Verification items for this drawing (mm, ordinates from the low corner). A direction names the side the tool comes from. Round coordinates to 2 decimals unless told otherwise and drop trailing zeros. Loops run counter-clockwise (first coordinate to the right, second up) from the corner with the lowest first, then second, coordinate; pieces in that order, holes last. Notation, with made-up numbers: M 69.5,57.5 L 88.5,57.5 A12 ccw 88.5,76.5 Z; hole C 84,10 d9. An arc over 180 degrees is marked long. Use one line per item in the form item = value. Start each with the question number.
1. Set-up check for the marked faces 4, 5 and 6: record each of +Z, -Z, +X, -X, +Y, -Y from which the full face is reachable in a straight line by a thin tool's end or side.
2. Material ranges on line 1 (Y direction, x = 16, z = 1) (3 decimals); line 2 (Y direction, x = 12, z = 1.5) (3 decimals); line 3 (X direction, y = 18, z = 2.8), recorded low to high.
3. Go/stop test with flat-tipped pins: pin 1 (0.9 mm diameter, centred on x = 4.5, z = 1, fed in from -Y) (3 decimals); pin 2 (1.6 mm diameter, centred on y = 2, z = 1.5, fed in from -X) (3 decimals); pin 3 (1.6 mm diameter, centred on y = 2, z = 2.5, fed in from +X) (3 decimals). Record where each tip stops, or that it passes through.
4. Cross-section at D-D (x = 5). Record the boundary of the cut face in (y, z) (3 decimals).
5. Draft check along X on the marked faces 1, 2 and 3. Enter one of: pulls with the +X half, pulls with the -X half, needs draft (parallel to the pull), parting line crosses it, or undercut.
6. Cross-section at A-A (x = 16). Record the boundary of the cut face in (y, z) (3 decimals), then the cut area to 3 significant figures.
7. Cross-section at B-B (z = 1.25). Record the boundary of the cut face in (x, y) (3 decimals).
8. Cross-section at C-C (y = 21.25). Record the boundary of the cut face in (x, z).
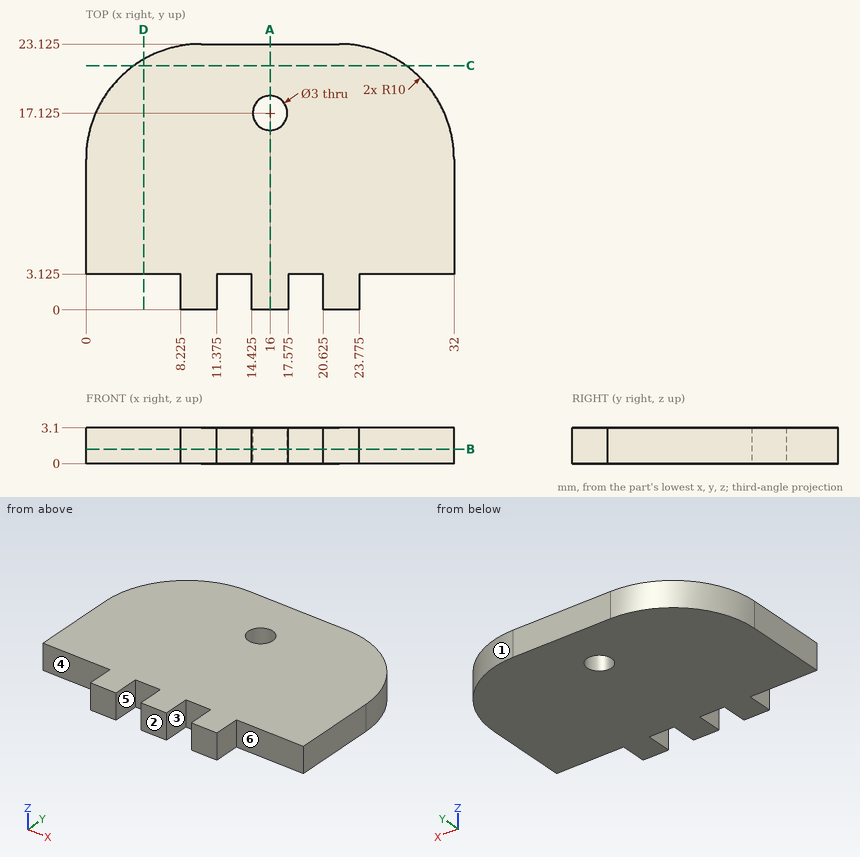
Reported:
q1.face_4 = +Z, -Z, -X, -Y
q1.face_5 = +Z, -Z, -Y
q1.face_6 = +Z, -Z, +X, -Y
q2.line_1 = 0 to 15.625, 18.625 to 23.125
q2.line_2 = 3.125 to 23.125
q2.line_3 = 1.27 to 14.78, 17.22 to 30.73
q3.pin_1 = 3.125
q3.pin_2 = 8.225
q3.pin_3 = 23.775
q4.outline = M 3.125,0 L 21.785,0 L 21.785,3.1 L 3.125,3.1 Z
q5.face_1 = pulls with the +X half
q5.face_2 = needs draft
q5.face_3 = undercut
q6.outline = M 0,0 L 15.625,0 L 15.625,3.1 L 0,3.1 Z; M 18.625,0 L 23.125,0 L 23.125,3.1 L 18.625,3.1 Z
q6.area = 62.4 mm²
q7.outline = M 0,3.125 L 8.225,3.125 L 8.225,0 L 11.375,0 L 11.375,3.125 L 14.425,3.125 L 14.425,0 L 17.575,0 L 17.575,3.125 L 20.625,3.125 L 20.625,0 L 23.775,0 L 23.775,3.125 L 32,3.125 L 32,13.125 A10 ccw 22,23.125 L 10,23.125 A10 ccw 0,13.125 Z; hole C 16,17.125 d3
q8.outline = M 4.17,0 L 27.83,0 L 27.83,3.1 L 4.17,3.1 Z
